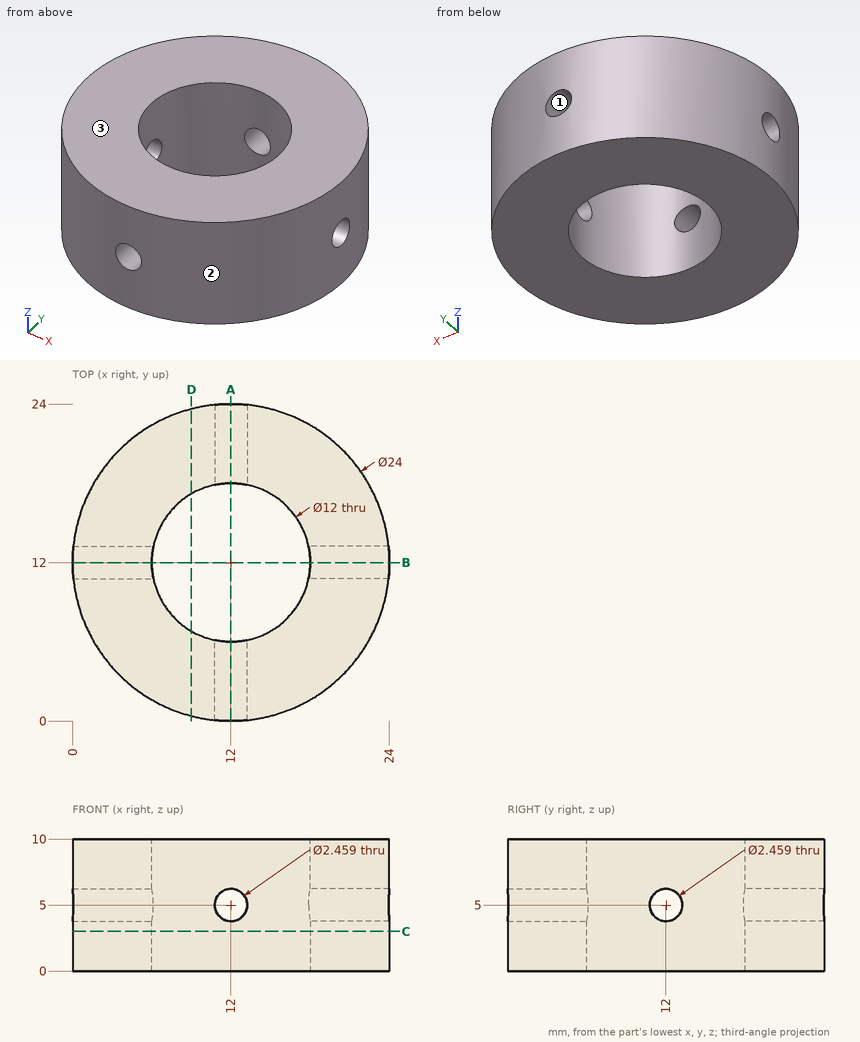
Drawing for the job (mm, zero at the part's lowest x, y, z). Coordinates: 2 decimals unless noted, no trailing zeros. Order: outer loops, then holes, each group sorted by start corner. A loop starts at its lowest first (then second) coordinate and runs counter-clockwise, first axis right, second up.
Item 1: Two-plate mould, pull along X, no slides. Class the marked faces 1, 2 and 3: +X half, -X half, draft (parallel to the pull), parting line (faces both ways), or undercut.
Check sheet entries:
face 1: undercut
face 2: parting line
face 3: draft
Item 2: Band-saw the part on C-C on z = 3. List the corners of the cut face in (x, y).
Check sheet entries:
outline: circle Ø24 at (12, 12); hole circle Ø12 at (12, 12)
Item 3: Pin check, flat tips, straight feed: pin 1 Ø2 at (y, z) = (16, 4.5) entering from +X; pin 2 Ø2 at (x, z) = (20, 7.5) entering from +Y. Stop position of each tip, or through.
Check sheet entries:
pin 1: stops at x = 23.62
pin 2: stops at y = 21.75
Item 4: Band-saw the part on D-D on x = 9. List the corners of the cut face in (y, z), plus the area to 3 significant figures.
Check sheet entries:
outline: (0.38, 0) - (6.8, 0) - (6.8, 10) - (0.38, 10) - close; (17.2, 0) - (23.62, 0) - (23.62, 10) - (17.2, 10) - close
area: 128 mm2
Item 5: Drill centre lines: L1, parallel to X at y = 16.75, z = 2.75; L2, parallel to X at y = 21.5, z = 4.75; L3, parallel to Y at x = 3, z = 5.25. Where is each one in solid material? Low to high.
Check sheet entries:
L1: x = 0.98 to 8.33, 15.67 to 23.02
L2: x = 4.67 to 10.8, 13.2 to 19.33
L3: y = 4.06 to 10.8, 13.2 to 19.94
Item 6: Band-saw the part on A-A on x = 12. List the corners of the cut face in (y, z).
Check sheet entries:
outline: (0, 0) - (6, 0) - (6, 3.77) - (0, 3.77) - close; (0, 6.23) - (6, 6.23) - (6, 10) - (0, 10) - close; (18, 0) - (24, 0) - (24, 3.77) - (18, 3.77) - close; (18, 6.23) - (24, 6.23) - (24, 10) - (18, 10) - close
